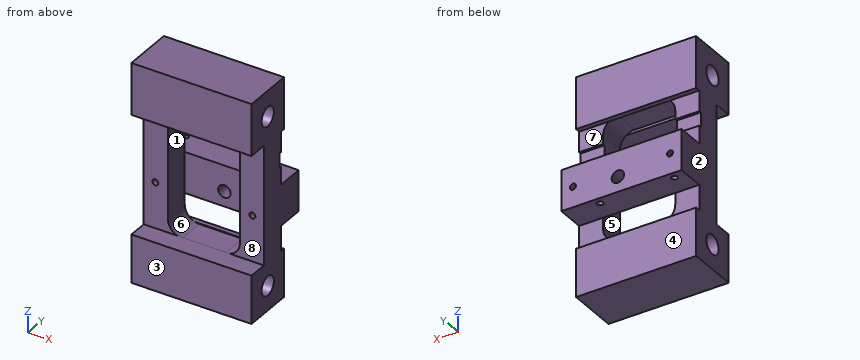
```python
from build123d import *

# Parameters (mm, degrees)
BOSS_EXTRUDE1_DEPTH            = 50
CUT_EXTRUDE1_REACH             = 108.241
M3_TAPPED_HOLE1_D              = 2.5
M3_TAPPED_HOLE2_D              = 2.5
SKETCH7_R                      = 2.577157182
CUT_EXTRUDE2_DEPTH             = 109.218528913
CUT_EXTRUDE3_REACH             = 110.219
SKETCH8_R                      = 4
CUT_EXTRUDE3_DIRECTION_2_DEPTH = 109.218528913


with BuildPart() as part:
    # Sketch1 → Boss-Extrude1 (new body)
    with BuildSketch(Plane(origin=(0, 0, 0), x_dir=(0, 0, -1), z_dir=(1, 0, 0))):
        Polygon((0, 0), (0, 21), (21.5, 21), (21.5, 19), (30, 19), (30, 18), (36, 18), (36, 19), (43.5, 19), (43.5, 30.5), (60.5, 30.5), (60.5, 19), (71, 19), (71, 21), (91, 21), (91, 0), (71, 0), (71, 8), (21.5, 8), (21.5, 0), align=None)
    extrude(amount=BOSS_EXTRUDE1_DEPTH)

    # Cut-Extrude1: up to this face of the body (flat: up to its plane)
    cut_extrude1_end = Plane(part.part.faces().sort_by_distance((25, 19, -65.75))[0])
    # Sketch2 → Cut-Extrude1 (cut, up to the picked face)
    with BuildSketch(Plane(origin=(0, 8, 0), x_dir=(1, 0, 0), z_dir=(0, 1, 0)), mode=Mode.PRIVATE) as cut_extrude1_sk1:
        with BuildLine():
            Line((16, 71.3), (34, 71.3))
            ThreePointArc((34, 71.3), (38.242640687, 69.542640687), (40, 65.3))
            Line((40, 65.3), (40, 26.3))
            ThreePointArc((40, 26.3), (38.242640687, 22.057359313), (34, 20.3))
            Line((34, 20.3), (16, 20.3))
            ThreePointArc((16, 20.3), (11.757359313, 22.057359313), (10, 26.3))
            Line((10, 26.3), (10, 65.3))
            ThreePointArc((10, 65.3), (11.757359313, 69.542640687), (16, 71.3))
        make_face()
    cut_extrude1_tool1 = split(extrude(cut_extrude1_sk1.sketch, amount=CUT_EXTRUDE1_REACH, mode=Mode.PRIVATE), bisect_by=cut_extrude1_end, keep=Keep.BOTH, mode=Mode.PRIVATE)
    add(cut_extrude1_tool1.solids().sort_by(Axis((25, 8, -45.8), (0, 1, 0)))[0], mode=Mode.SUBTRACT)

    # M3 Tapped Hole1 (through all)
    with Locations(Plane(origin=(0, 30.5, 0), x_dir=(1, 0, 0), z_dir=(0, 1, 0))):
        with Locations((4.8, 52), (45.2, 52)):
            Hole(M3_TAPPED_HOLE1_D / 2)

    # M3 Tapped Hole2 (through all)
    with Locations(Plane(origin=(0, 0, -60.5), x_dir=(-1, 0, 0), z_dir=(0, 0, -1))):
        with Locations((-4.8, 27.5), (-35.8, 27.5)):
            Hole(M3_TAPPED_HOLE2_D / 2)

    # Sketch7 → Cut-Extrude2 (cut, through all)
    with BuildSketch(Plane(origin=(0, 30.5, 0), x_dir=(1, 0, 0), z_dir=(0, 1, 0))):
        with Locations(Location((26.5, 54.2, 0), (0, 0, 270))):
            Circle(SKETCH7_R)
    extrude(amount=-CUT_EXTRUDE2_DEPTH, mode=Mode.SUBTRACT)

    # Sketch8 → Cut-Extrude3 (cut, up to next)
    with BuildSketch(Plane(origin=(50, 0, 0), x_dir=(0, 0, -1), z_dir=(1, 0, 0)), mode=Mode.PRIVATE) as cut_extrude3_sk1:
        with Locations(Location((10.75, 10.5, 0), (0, 0, 180))):
            Circle(SKETCH8_R)
    cut_extrude3_tool1 = extrude(cut_extrude3_sk1.sketch, amount=-CUT_EXTRUDE3_REACH, mode=Mode.PRIVATE) & part.part
    # Sketch8 → Cut-Extrude3 (cut, up to next)
    with BuildSketch(Plane(origin=(50, 0, 0), x_dir=(0, 0, -1), z_dir=(1, 0, 0)), mode=Mode.PRIVATE) as cut_extrude3_sk2:
        with Locations(Location((80.75, 10.5, 0), (0, 0, 180))):
            Circle(SKETCH8_R)
    cut_extrude3_tool2 = extrude(cut_extrude3_sk2.sketch, amount=-CUT_EXTRUDE3_REACH, mode=Mode.PRIVATE) & part.part
    add(cut_extrude3_tool1.solids().sort_by_distance((50, 10.5, -10.75))[0], mode=Mode.SUBTRACT)
    add(cut_extrude3_tool2.solids().sort_by_distance((50, 10.5, -80.75))[0], mode=Mode.SUBTRACT)

    # Sketch8 → Cut-Extrude3 direction 2 (cut)
    with BuildSketch(Plane(origin=(50, 0, 0), x_dir=(0, 0, -1), z_dir=(1, 0, 0))):
        with Locations(Location((10.75, 10.5, 0), (0, 0, 180))):
            Circle(SKETCH8_R)
        with Locations(Location((80.75, 10.5, 0), (0, 0, 180))):
            Circle(SKETCH8_R)
    extrude(amount=CUT_EXTRUDE3_DIRECTION_2_DEPTH, mode=Mode.SUBTRACT)


solid = part.part
```
Check sheet for the modelled part. Datum: model origin and axes. Units: mm. Face numbers are marked on the shaded views. A direction names the side the tool comes from. Give positions to 0.01 mm unless a question says otherwise; leave off trailing zeros. Loops run counter-clockwise (first coordinate to the right, second up) from the corner with the lowest first, then second, coordinate; pieces in that order, holes last. Notation, with made-up numbers: (72, -1.75) - (77, -1.75) arc R28 ccw to (77, 19.25) - close; hole circle Ø10 at (33.5, 72.25). An arc over 180 degrees is marked (long way). One line per question, with ' | ' between items. Start each with the question number.
1. Cross-section at B-B, the plane x = 4.8. Give the number of separate pieces and of enclosed holes in the cut face, plus the area to 3 significant figures.
2. Gauge pin test, flat ends, axial feed: pin 1 Ø15.5 at (x, z) = (10, -48) entering from -Y; pin 2 Ø8 at (y, z) = (14, -54.5) entering from -X; pin 3 Ø2.5 at (x, z) = (6, -26.5) entering from +Y; pin 4 Ø3 at (x, y) = (4.8, 27.5) entering from -Z. Record the tip position at first contact, or that the pin passes through.
3. Draft check along X on the marked faces 1, 2 and 3. Enter one of: released by +X, released by -X, zero draft, split by the parting line, or undercut.
4. Cross-section at C-C, the plane x = 45.2. Enter the section's corners in (y, z), plus the area to 3 significant figures.
5. Material ranges on line 1 along X through (y, z) = (18.5, -52); line 2 along Z through (x, y) = (14.5, 19.5); line 3 along Z through (x, y) = (8, 10.5), recorded low to high. Write a range as [from, to].
6. Cross-section at D-D, the plane x = 30. Enter the section's corners in (y, z).
7. Cross-section at A-A, the plane z = -54.2. Enter the section's corners in (x, y).
8. Set-up check for the marked faces 4, 5, 6, 7 and 8: record each of +Z, -Z, +X, -X, +Y, -Y from which the full face is reachable in a straight line by a thin tool's end or side.
Check result:
1) separate pieces: 4 | enclosed holes: 2 | area: 1,410 mm2
2) pin 1: stops at y = 8 | pin 2: stops at x = 0 | pin 3: stops at y = 19 | pin 4: stops at z = -60.5
3) face 1: undercut | face 2: released by -X | face 3: zero draft
4) outline: (0, -91) - (21, -91) - (21, -71) - (19, -71) - (19, -60.5) - (30.5, -60.5) - (30.5, -53.25) - (8, -53.25) - (8, -71) - (0, -71) - close; (0, -21.5) - (8, -21.5) - (8, -50.75) - (30.5, -50.75) - (30.5, -43.5) - (19, -43.5) - (19, -36) - (18, -36) - (18, -30) - (19, -30) - (19, -21.5) - (21, -21.5) - (21, 0) - (0, 0) - close; hole circle Ø8 at (10.5, -80.75); hole circle Ø8 at (10.5, -10.75) | area: 1,450 mm2
5) line 1: x = [0, 3.55], [6.05, 10], [40, 43.95], [46.45, 50] | line 2: z = [-91, -71], [-60.5, -43.5], [-21.5, 0] | line 3: z = [-91, -84.75], [-76.75, -14.75], [-6.75, 0]
6) outline: (0, -91) - (21, -91) - (21, -71) - (19, -71) - (19, -71.3) - (8, -71.3) - (8, -71) - (0, -71) - close; (0, -21.5) - (8, -21.5) - (8, -20.3) - (19, -20.3) - (19, -21.5) - (21, -21.5) - (21, 0) - (0, 0) - close; (19, -60.5) - (30.5, -60.5) - (30.5, -43.5) - (19, -43.5) - close; hole circle Ø8 at (10.5, -80.75); hole circle Ø8 at (10.5, -10.75)
7) outline: (0, 8) - (10, 8) - (10, 19) - (23.92, 19) - (23.92, 30.5) - (0, 30.5) - close; (29.08, 19) - (40, 19) - (40, 8) - (50, 8) - (50, 30.5) - (29.08, 30.5) - close; hole circle Ø2.5 at (4.8, 27.5); hole circle Ø2.5 at (35.8, 27.5)
8) face 4: -Z, +X, -X, +Y | face 5: -Y | face 6: none | face 7: +X, -X, +Y | face 8: +X, -X, -Y
